Autodesk Inventor part; units mm, degrees
ref_plane "plate_rivet_XY" through (0, 0, 0) normal (0, -1, 0) x (1, 0, 0)
ref_plane "plate_rivet_YZ" through (0, 0, 0) normal (1, 0, 0) x (0, 0, 1)
ref_plane "plate_rivet_ZX" through (0, 0, 0) normal (0, 0, 1) x (0, -1, 0)
sketch "Sketch_1" plane through (0, 0, 0) normal (0, 0, 1) x (1, 0, 0)
  line L0 (0, -13.5382) -> (0, 4.4704)
  line L1 (0, 4.4704) -> (9.144, 4.4704)
  arc A0 (9.9314, 3.683) -> (9.144, 4.4704) centre (9.144, 3.683) ccw
  line L2 (9.9314, 3.683) -> (9.9314, 0.7874)
  arc A1 (9.144, 0) -> (9.9314, 0.7874) centre (9.144, 0.7874) ccw
  line L3 (9.144, 0) -> (6.6802, 0)
  arc A2 (6.6802, 0) -> (6.2738, -0.4064) centre (6.6802, -0.4064) ccw
  line L4 (6.2738, -0.4064) -> (6.2738, -11.1506)
  line L5 (6.2738, -11.1506) -> (6.8199, -11.1506)
  arc A3 (6.8199, -13.5382) -> (6.8199, -11.1506) centre (6.8199, -12.3444) ccw
  line L6 (6.8199, -13.5382) -> (0, -13.5382)
  line L7 (0, -13.5382) -> (0, 4.4704)
revolve "Revolution1" add sketch "Sketch_1" angle 360 about axis through (0, -13.5382, 0) along (0, -1, 0)
ref_plane "plate_rivet_XY" through (0, 0, 0) normal (0, -1, 0) x (1, 0, 0)
ref_plane "plate_rivet_YZ" through (0, 0, 0) normal (1, 0, 0) x (0, 0, 1)
ref_plane "plate_rivet_ZX" through (0, 0, 0) normal (0, 0, 1) x (0, -1, 0)
properties part number "2SS-R"
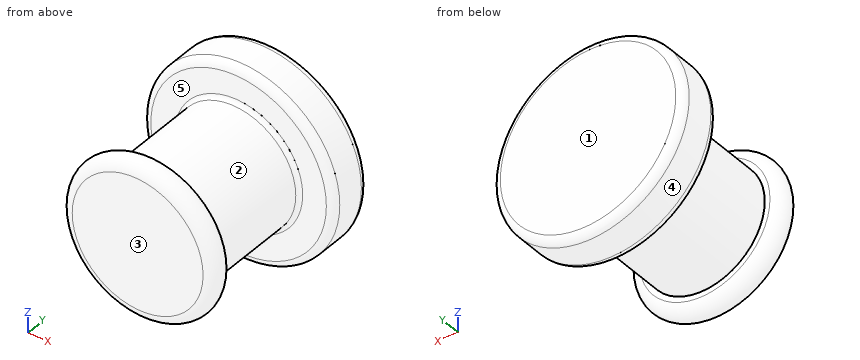
Could you check a few things on this model? Use its own coordinates, in mm. Face numbers are marked on the shaded views. A direction names the side the tool comes from. Round coordinates to 2 decimals unless told otherwise and drop trailing zeros. Loops run counter-clockwise (first coordinate to the right, second up) from the corner with the lowest first, then second, coordinate; pieces in that order, holes last.
Q1. For P1, Ø1, axis at y = -5, z = 5.5, coming from the -X side; P2, Ø3, axis at x = -5, y = -3.5, coming from the +Z side; P3, Ø5, axis at x = -5, y = -10, coming from the +Z side, each with a flat end and sliding along its axis, tell me the tip position at first contact or that it passes through.
Q2. I want a section at C-C (y = -8.25). Write out the boundary of the cut face in (x, z).
Q3. I want a section at A-A (z = 0). Write out the boundary of the cut face in (x, y), and give its area (3 significant figures).
Q4. On a 3-axis mill with a long thin cutter (end or side, diameter ignored), from which of +Z, -Z, +X, -X, +Y, -Y can I reach the whole of each face in a straight line? I mean the marked faces 4 and 5. Say none if no direction works.
Q5. I want a section at B-B (x = 0). Write out the boundary of the cut face in (y, z), and give its area (3 significant figures).
Q6. Thinking about a two-plate mould opening in Y: for the marked faces 1, 2 and 3, which applies, pulls with the +Y half, pulls with the -Y half, needs draft (parallel to the pull), parting line crosses it, or undercut?
Q7. Please list where these lines run through material, in increasing order: L1, parallel to Z at x = 0.25, y = -4.25; L2, parallel to Y at x = -3.25, z = 8.5; L3, parallel to X at y = 3.5, z = -0.25.
Answer below:
1. P1: stops at x = -3.79
1. P2: stops at z = 5.21
1. P3: stops at z = 7.18
2. outline: circle Ø12.55 at (0, 0)
3. outline: (-9.93, 0.79) arc R0.79 ccw to (-9.14, 0) - (-6.68, 0) arc R0.41 cw to (-6.27, -0.41) - (-6.27, -11.15) - (-6.82, -11.15) arc R1.19 ccw to (-6.82, -13.54) - (6.82, -13.54) arc R1.19 ccw to (6.82, -11.15) - (6.27, -11.15) - (6.27, -0.41) arc R0.41 cw to (6.68, 0) - (9.14, 0) arc R0.79 ccw to (9.93, 0.79) - (9.93, 3.68) arc R0.79 ccw to (9.14, 4.47) - (-9.14, 4.47) arc R0.79 ccw to (-9.93, 3.68) - close
3. area: 265 mm2
4. face 4: +Y, -Y
4. face 5: none
5. outline: (-13.54, -6.82) arc R1.19 ccw to (-11.15, -6.82) - (-11.15, -6.27) - (-0.41, -6.27) arc R0.41 cw to (0, -6.68) - (0, -9.14) arc R0.79 ccw to (0.79, -9.93) - (3.68, -9.93) arc R0.79 ccw to (4.47, -9.14) - (4.47, 9.14) arc R0.79 ccw to (3.68, 9.93) - (0.79, 9.93) arc R0.79 ccw to (0, 9.14) - (0, 6.68) arc R0.41 cw to (-0.41, 6.27) - (-11.15, 6.27) - (-11.15, 6.82) arc R1.19 ccw to (-13.54, 6.82) - close
5. area: 265 mm2
6. face 1: pulls with the +Y half
6. face 2: undercut
6. face 3: pulls with the -Y half
7. L1: z = -6.27 to 6.27
7. L2: y = 0 to 4.47
7. L3: x = -9.93 to 9.93
